Could you check a few things on this model? Use its own coordinates, in mm. Give positions to 0.01 mm unless a question says otherwise; leave off trailing zeros. Write each loop counter-clockwise with the first axis right and the second up, starting at its lowest first coordinate (ties: lowest second). Pieces come first, ordered by that corner, then holes. Notation, with made-up numbers: (70.25, 75.25) - (120.25, 75.25) arc R38 ccw to (120.25, 113.25) - close; hole circle Ø6 at (29.5, 43). An arc over 180 degrees is marked (long way). Answer as CSV lines item,"result". Start each with the question number.
Q1. Imagine slicing it at A-A on z = 1.65. List the corners of the cut face in (x, y) for me, and give its area (3 significant figures).
Q2. Imagine slicing it at C-C on y = -12. List the corners of the cut face in (x, z) for me, and give its area (3 significant figures).
Q3. If I drill on line 1 along Y through (x, z) = (-43, 0.45); line 2 along X through (y, z) = (9, 3.3); line 3 along X through (y, z) = (-7, 1.7), over which ranges is the centre line in solid material (lowest first)?
Q4. Will these pins go through, and if not, where does the flat tip stop? pin 1 Ø1.5 at (x, z) = (-13, 2.5) entering from +Y; pin 2 Ø1 at (x, z) = (-64, 1.5) entering from -Y.
Q5. Imagine slicing it at B-B on x = 13. List the corners of the cut face in (y, z) for me, and give its area (3 significant figures).
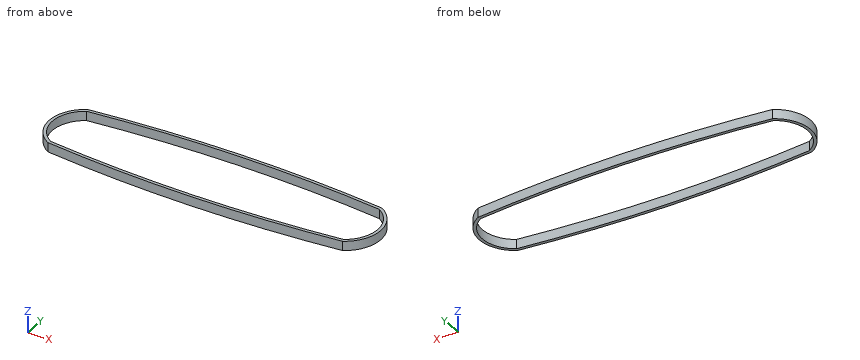
```python
from build123d import *

# Parameters (mm, degrees)
F1_DEPTH = 4.9


with BuildPart() as f1:
    # F0 (on Top) → F1 (new body)
    with BuildSketch(Plane.XY):
        with BuildLine():
            ThreePointArc((30.528466, -22.028455), (40.097824, -5.476208), (30.528466, 11.076038))
            ThreePointArc((30.528466, 11.076038), (-47.488298, 15.427198), (-125.505062, 11.076038))
            ThreePointArc((-125.505062, 11.076038), (-135.07442, -5.476208), (-125.505062, -22.028455))
            ThreePointArc((-125.505062, -22.028455), (-47.488298, -26.379615), (30.528466, -22.028455))
        make_face()
        with BuildLine():
            ThreePointArc((-124.988298, -20.476208), (-133.47442, -5.476208), (-124.988298, 9.523792))
            ThreePointArc((-124.988298, 9.523792), (-47.488298, 13.827198), (30.011702, 9.523792))
            ThreePointArc((30.011702, 9.523792), (38.497824, -5.476208), (30.011702, -20.476208))
            ThreePointArc((30.011702, -20.476208), (-47.488298, -24.779615), (-124.988298, -20.476208))
        make_face(mode=Mode.SUBTRACT)
    extrude(amount=F1_DEPTH)


solid = f1.part
```
Conclusion:
1,outline,"(-125.51, -22.03) arc R701.6 ccw to (30.53, -22.03) arc R19.1 ccw to (30.53, 11.08) arc R701.6 ccw to (-125.51, 11.08) arc R19.1 ccw to start; hole (-124.99, -20.48) arc R700 ccw to (30.01, -20.48) arc R17.5 ccw to (30.01, 9.52) arc R700 ccw to (-124.99, 9.52) arc R17.5 ccw to start"
1,area,"620 mm^2"
2,outline,"(-133.93, 0) - (-132.21, 0) - (-132.21, 4.9) - (-133.93, 4.9) - close; (37.24, 0) - (38.95, 0) - (38.95, 4.9) - (37.24, 4.9) - close"
2,area,"16.8 mm^2"
3,line 1,"-26.37 to -24.77, 13.81 to 15.41"
3,line 2,"-128.43 to -125.81, 30.83 to 33.46"
3,line 3,"-135.01 to -133.41, 38.43 to 40.04"
4,pin 1,"y = 14.62"
4,pin 2,"y = -26.2"
5,outline,"(-23.77, 0) - (-22.16, 0) - (-22.16, 4.9) - (-23.77, 4.9) - close; (11.21, 0) - (12.81, 0) - (12.81, 4.9) - (11.21, 4.9) - close"
5,area,"15.7 mm^2"
